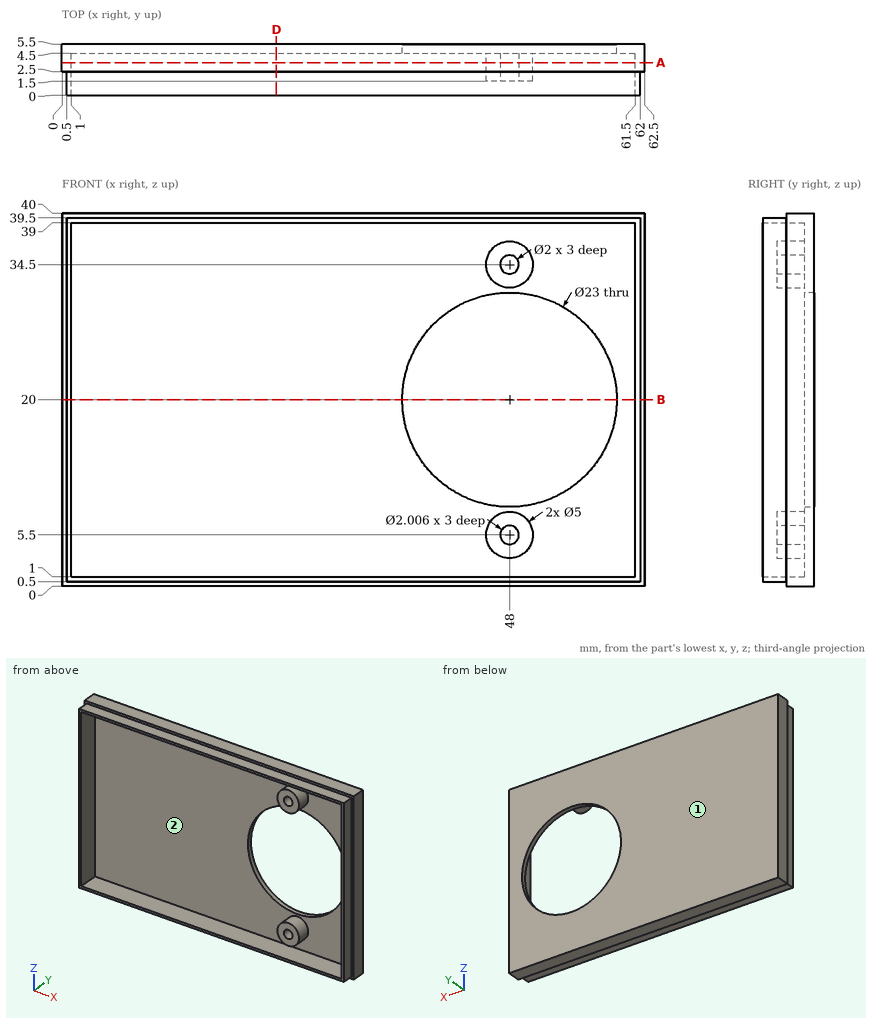
Print and shaded views of the part. All mm, measured from the part's lowest x, y and z. Coordinates: 2 decimals unless noted, no trailing zeros. Order: outer loops, then holes, each group sorted by start corner. A loop starts at its lowest first (then second) coordinate and runs counter-clockwise, first axis right, second up.
Item 1: Mould opens along X. For the marked faces 1 and 2 say: released by +X, released by -X, zero draft, split by the parting line, or undercut.
Filled in:
face 1: zero draft
face 2: undercut
Item 2: Saw through at B-B on z = 20. List the corners of the cut face in (x, y).
Filled in:
outline: (0, 2.5) - (0.5, 2.5) - (0.5, 0) - (1, 0) - (1, 4.5) - (36.5, 4.5) - (36.5, 5.5) - (0, 5.5) - close; (59.5, 4.5) - (61.5, 4.5) - (61.5, 0) - (62, 0) - (62, 2.5) - (62.5, 2.5) - (62.5, 5.5) - (59.5, 5.5) - close
Item 3: Saw through at A-A on y = 3.5. List the corners of the cut face in (x, z), then the cut area to 3 significant figures.
Filled in:
outline: (0, 0) - (62.5, 0) - (62.5, 40) - (0, 40) - close; circle Ø5 at (48, 5.5); circle Ø5 at (48, 34.5); hole (1, 1) - (61.5, 1) - (61.5, 39) - (1, 39) - close; hole circle Ø2.01 at (48, 5.5); hole circle Ø2 at (48, 34.5)
area: 234 mm2
Item 4: Drop flat-ended pins along their axis: pin 1 Ø20 at (x, z) = (46, 15.5) entering from -Y; pin 2 Ø12 at (x, z) = (13, 29) entering from -Y; pin 3 Ø14 at (x, z) = (48, 20) entering from -Y; pin 4 Ø0.8 at (x, y) = (38, 2) entering from +Z. Give the stop position or say it passes through.
Filled in:
pin 1: stops at y = 1.5
pin 2: stops at y = 4.5
pin 3: passes through
pin 4: stops at z = 39.5
Item 5: Drill centre lines: L1, parallel to X at y = 3.45, z = 5.5; L2, parallel to Z at x = 48, y = 2.55; L3, parallel to Z at x = 57.5, y = 1.4. Where is each one in solid material? Low to high.
Filled in:
L1: x = 0 to 1, 45.5 to 47, 49 to 50.5, 61.5 to 62.5
L2: z = 0 to 1, 3 to 4.5, 6.5 to 8, 32 to 33.5, 35.5 to 37, 39 to 40
L3: z = 0.5 to 1, 39 to 39.5
Item 6: Saw through at D-D on x = 23. List the corners of the cut face in (y, z).
Filled in:
outline: (0, 0.5) - (2.5, 0.5) - (2.5, 0) - (5.5, 0) - (5.5, 40) - (2.5, 40) - (2.5, 39.5) - (0, 39.5) - (0, 39) - (4.5, 39) - (4.5, 1) - (0, 1) - close
